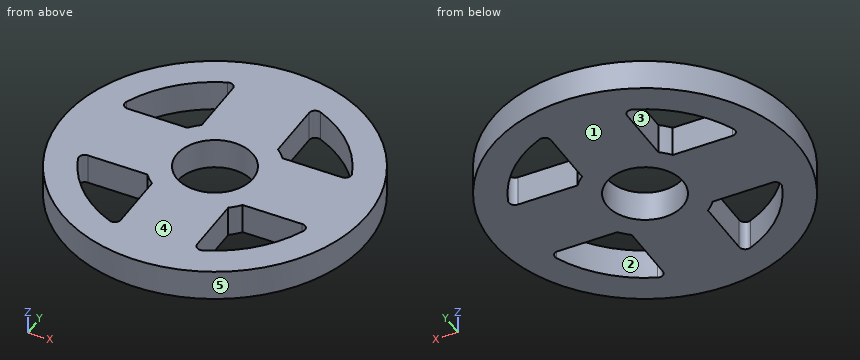
from build123d import *

# Parameters (mm, degrees)
SKETCH1_R           = 25
SKETCH1_R_2         = 10
SKETCH1_R_3         = 6.25
BOSS_EXTRUDE1_DEPTH = 5


with BuildPart() as part:
    # Sketch1 → Boss-Extrude1 (new body)
    # profile 1 of 2: a face of its own
    with BuildSketch(Plane.XY):
        Circle(SKETCH1_R)
        with BuildLine():
            Line((17.56238879, 6.25), (7.806247498, 6.25))
            ThreePointArc((7.806247498, 6.25), (9.43563657, 3.311912214), (10, 0))
            ThreePointArc((10, 0), (9.43563657, -3.311912214), (7.806247498, -6.25))
            Line((7.806247498, -6.25), (17.56238879, -6.25))
            ThreePointArc((17.56238879, -6.25), (18.393526247, -6.693932984), (18.486725042, -7.631578947))
            ThreePointArc((18.486725042, -7.631578947), (14.142135624, -14.142135624), (7.631578947, -18.486725042))
            ThreePointArc((7.631578947, -18.486725042), (6.693932984, -18.393526247), (6.25, -17.56238879))
            Line((6.25, -17.56238879), (6.25, -7.806247498))
            ThreePointArc((6.25, -7.806247498), (0, -10), (-6.25, -7.806247498))
            Line((-6.25, -7.806247498), (-6.25, -17.56238879))
            ThreePointArc((-6.25, -17.56238879), (-6.693932984, -18.393526247), (-7.631578947, -18.486725042))
            ThreePointArc((-7.631578947, -18.486725042), (-14.142135624, -14.142135624), (-18.486725042, -7.631578947))
            ThreePointArc((-18.486725042, -7.631578947), (-18.393526247, -6.693932984), (-17.56238879, -6.25))
            Line((-17.56238879, -6.25), (-7.806247498, -6.25))
            ThreePointArc((-7.806247498, -6.25), (-10, 0), (-7.806247498, 6.25))
            Line((-7.806247498, 6.25), (-17.56238879, 6.25))
            ThreePointArc((-17.56238879, 6.25), (-18.393526247, 6.693932984), (-18.486725042, 7.631578947))
            ThreePointArc((-18.486725042, 7.631578947), (-14.142135624, 14.142135624), (-7.631578947, 18.486725042))
            ThreePointArc((-7.631578947, 18.486725042), (-6.693932984, 18.393526247), (-6.25, 17.56238879))
            Line((-6.25, 17.56238879), (-6.25, 7.806247498))
            ThreePointArc((-6.25, 7.806247498), (0, 10), (6.25, 7.806247498))
            Line((6.25, 7.806247498), (6.25, 17.56238879))
            ThreePointArc((6.25, 17.56238879), (6.693932984, 18.393526247), (7.631578947, 18.486725042))
            ThreePointArc((7.631578947, 18.486725042), (14.142135624, 14.142135624), (18.486725042, 7.631578947))
            ThreePointArc((18.486725042, 7.631578947), (18.393526247, 6.693932984), (17.56238879, 6.25))
        make_face(mode=Mode.SUBTRACT)
    # profile 2 of 2: a face of its own
    with BuildSketch(Plane.XY):
        Circle(SKETCH1_R_2)
        Circle(SKETCH1_R_3, mode=Mode.SUBTRACT)
    extrude(amount=BOSS_EXTRUDE1_DEPTH)


solid = part.part
For this review, take the finished solid that the model builds, in its own axes (mm). Face numbers are marked on the shaded views. A direction names the side the tool comes from. Round coordinates to 2 decimals unless told otherwise and drop trailing zeros. Order: outer loops, then holes, each group sorted by start corner. A loop starts at its lowest first (then second) coordinate and runs counter-clockwise, first axis right, second up. Notation, with made-up numbers: (84.25, 13) -> (112.25, 13) arc R18 ccw to (112.25, 26) -> close; hole circle Ø1 at (-33, 87). An arc over 180 degrees is marked (long way). Write item = value, one per line. Start each with the question number.
1) Take a section at B-B on y = -12. State the section outline as (x, z) points.
2) Take a section at A-A on x = 0. State the section outline as (y, z) points.
3) To check wall thickness, follow line 1 (Y direction, x = 0, z = 4.05); line 2 (Y direction, x = -9, z = 3.9); line 3 (X direction, y = 7, z = 1.45). State the ranges of each line that lie inside material, in increasing order. Write a range as from..to.
4) Tool access review of the marked faces 1 and 2: name each direction out of +Z, -Z, +X, -X, +Y, -Y from which nothing blocks a thin tool from reaching the whole face with its end or side.
5) Take a section at D-D on z = 3.55. State the section outline as (x, y) points.
6) Insertion check: pin 1 (2.5 mm diameter, centred on x = 13.5, z = 2.5, fed in from +Y); pin 2 (2.5 mm diameter, centred on x = -12.5, z = 1.5, fed in from -Y); pin 3 (2.5 mm diameter, centred on x = -12, z = 1.5, fed in from +Y). Each pin has a flat end and moves straight along its axis. Give the tip position at first contact, or say it passes through.
7) The part is to be moulded in two halves that separate along X. For the marked faces 3, 4 and 5, say which applies: +X half, -X half, draft (parallel to the pull), parting line (faces both ways), or undercut.
Verdict:
q1.outline = (-21.93, 0) -> (-16, 0) -> (-16, 5) -> (-21.93, 5) -> close; (-6.25, 0) -> (6.25, 0) -> (6.25, 5) -> (-6.25, 5) -> close; (16, 0) -> (21.93, 0) -> (21.93, 5) -> (16, 5) -> close
q2.outline = (-25, 0) -> (-6.25, 0) -> (-6.25, 5) -> (-25, 5) -> close; (6.25, 0) -> (25, 0) -> (25, 5) -> (6.25, 5) -> close
q3.line_1 = -25..-6.25, 6.25..25
q3.line_2 = -23.32..-17.86, -6.25..6.25, 17.86..23.32
q3.line_3 = -24..-18.53, -7.14..7.14, 18.53..24
q4.face_1 = -Z, +X, -X, +Y, -Y
q4.face_2 = +Z, -Z
q5.outline = circle Ø50 at (0, 0); hole (-18.49, -7.63) arc R20 ccw to (-7.63, -18.49) arc R1 ccw to (-6.25, -17.56) -> (-6.25, -7.81) arc R10 cw to (-7.81, -6.25) -> (-17.56, -6.25) arc R1 ccw to start; hole (-18.49, 7.63) arc R1 ccw to (-17.56, 6.25) -> (-7.81, 6.25) arc R10 cw to (-6.25, 7.81) -> (-6.25, 17.56) arc R1 ccw to (-7.63, 18.49) arc R20 ccw to start; hole circle Ø12.5 at (0, 0); hole (6.25, -17.56) arc R1 ccw to (7.63, -18.49) arc R20 ccw to (18.49, -7.63) arc R1 ccw to (17.56, -6.25) -> (7.81, -6.25) arc R10 cw to (6.25, -7.81) -> close; hole (6.25, 7.81) arc R10 cw to (7.81, 6.25) -> (17.56, 6.25) arc R1 ccw to (18.49, 7.63) arc R20 ccw to (7.63, 18.49) arc R1 ccw to (6.25, 17.56) -> close
q6.pin_1 = 21.79
q6.pin_2 = -22.33
q6.pin_3 = 22.57
q7.face_3 = undercut
q7.face_4 = draft
q7.face_5 = parting line
